For this review, use the dimensioned drawing (mm, ordinates from the lowest corner) and the shaded views. A direction names the side the tool comes from. Coordinates: 2 decimals unless noted, no trailing zeros. Order: outer loops, then holes, each group sorted by start corner. A loop starts at its lowest first (then second) coordinate and runs counter-clockwise, first axis right, second up. Notation, with made-up numbers: (-16, -40) -> (20, -40) arc R19 cw to (20, -36) -> close; hole circle Ø11 at (18, 88). An arc over 180 degrees is marked (long way). Return JSON: item names as keys, results as strings. Group by question number.
Item 1: Machinability: for the marked faces 4 and 5, which of the approach directions +Z, -Z, +X, -X, +Y, -Y give a long, thin tool a straight path to every point of the face, cutting with its end or side? Answer none if there is none.
Item 2: Take a section at B-B (x = 88). Write out the cut boundary in (y, z).
Item 3: Take a section at A-A (y = 9.25). Write out the cut boundary in (x, z), then the cut area to 3 significant figures.
Item 4: Take a section at C-C (y = 20.75). Count the separate pieces of the cut face and the enclosed holes in it, then the cut area to 3 significant figures.
Item 5: Insertion check: pin 1 (3 mm diameter, centred on x = 143.32, z = 11.42, fed in from +Y). The pin has a flat end and moves straight along its axis. Give the tip position at first contact, or say it passes through.
Item 6: Draft analysis for pull direction Y (two halves, no side actions). For the marked faces 1, 2 and 3, state which applies: +Y half, -Y half, draft (parallel to the pull), parting line (faces both ways), or undercut.
Item 7: For line 1 along Z through (x, y) = (123, 22.25); line 2 along Y through (x, z) = (28, 7); line 3 along Z through (x, y) = (126, 5), list the stretches that pass through material, from the lowest coordinate up.
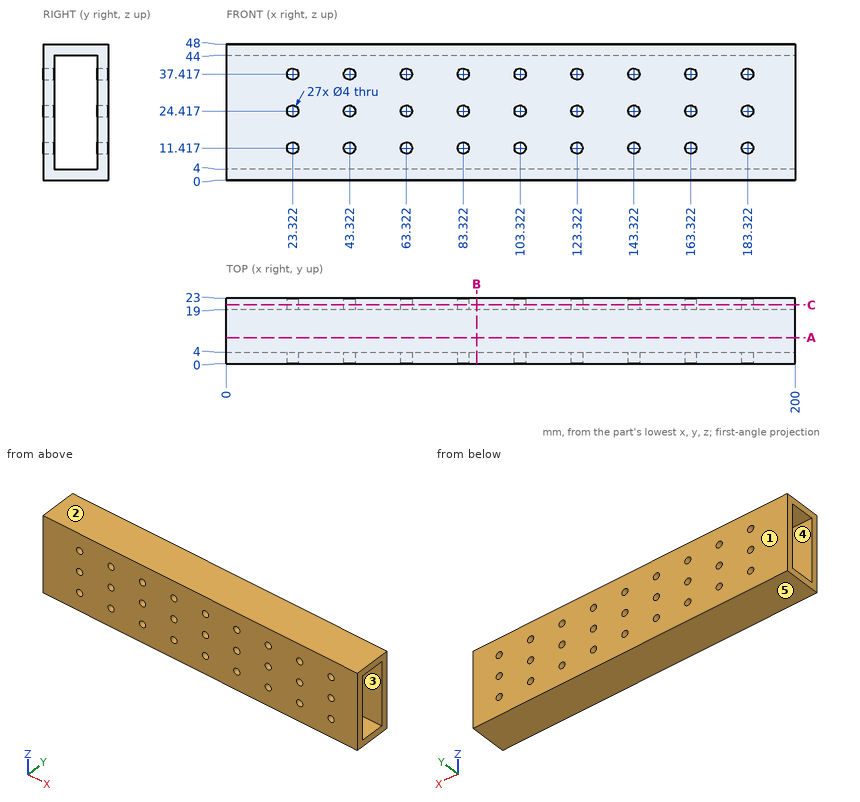
Findings below:
{
 "1": {"face 4": "+X, -X", "face 5": "-Z, +X, -X, +Y, -Y"},
 "2": {"outline": "(0, 0) -> (23, 0) -> (23, 48) -> (0, 48) -> close; hole (4, 4) -> (19, 4) -> (19, 44) -> (4, 44) -> close"},
 "3": {"outline": "(0, 0) -> (200, 0) -> (200, 4) -> (0, 4) -> close; (0, 44) -> (200, 44) -> (200, 48) -> (0, 48) -> close", "area": "1,600 mm2"},
 "4": {"separate pieces": "1", "enclosed holes": "27", "area": "9,260 mm2"},
 "5": {"pin 1": "passes through"},
 "6": {"face 1": "+Y half", "face 2": "draft", "face 3": "undercut"},
 "7": {"line 1": "z = 0 to 9.44, 13.39 to 22.44, 26.39 to 35.44, 39.39 to 48", "line 2": "y = 0 to 4, 19 to 23", "line 3": "z = 0 to 4, 44 to 48"}
}
